from build123d import *

# Parameters (mm, degrees)
ESBO_O1_R                = 62.5
ESBO_O1_R_2              = 4
RESSALTO_EXTRUS_O1_DEPTH = 20
ESBO_O2_R                = 38
RESSALTO_EXTRUS_O2_DEPTH = 35
ESBO_O4_R                = 12
CORTE_EXTRUS_O1_DEPTH    = 25


with BuildPart() as part:
    # Esboço1 → Ressalto-extrusão1 (new body)
    with BuildSketch(Plane(origin=(0, 0, 0), x_dir=(0, 0, -1), z_dir=(1, 0, 0))):
        Circle(ESBO_O1_R)
        with Locations((37.775, 30)):
            Circle(ESBO_O1_R_2, mode=Mode.SUBTRACT)
        with Locations((-37.775, 30)):
            Circle(ESBO_O1_R_2, mode=Mode.SUBTRACT)
        with Locations((37.775, -30)):
            Circle(ESBO_O1_R_2, mode=Mode.SUBTRACT)
        with Locations((-37.775, -30)):
            Circle(ESBO_O1_R_2, mode=Mode.SUBTRACT)
    extrude(amount=RESSALTO_EXTRUS_O1_DEPTH)

    # Esboço2 → Ressalto-extrusão2 (add)
    with BuildSketch(Plane(origin=(20, 0, 0), x_dir=(0, 0, -1), z_dir=(1, 0, 0))):
        Circle(ESBO_O2_R)
    extrude(amount=RESSALTO_EXTRUS_O2_DEPTH)

    # Esboço4 → Corte-extrusão1 (cut)
    with BuildSketch(Plane(origin=(55, 0, 0), x_dir=(0, 0, -1), z_dir=(1, 0, 0))):
        Circle(ESBO_O4_R)
    extrude(amount=-CORTE_EXTRUS_O1_DEPTH, mode=Mode.SUBTRACT)


solid = part.part
Design review of the part built by this model. Coordinates are the model's own, in mm. A direction names the side the tool comes from. Round coordinates to 2 decimals unless told otherwise and drop trailing zeros. Write each loop counter-clockwise with the first axis right and the second up, starting at its lowest first coordinate (ties: lowest second). Pieces come first, ordered by that corner, then holes.
Item 1: For pin 1 Ø5 at (x, z) = (43.5, -16.5) entering from +Y; pin 2 Ø3 at (x, z) = (41.5, -19.5) entering from -Y; pin 3 Ø10.5 at (y, z) = (30, 37.775) entering from +X; pin 4 Ø5 at (y, z) = (-30, -37.775) entering from +X, all flat-tipped, find the tip position at first contact; note any pin that passes through.
Item 2: Consider section B-B on z = 36.5. Give the boundary of the cut face in (x, y).
Item 3: Draft analysis for pull direction Y (two halves, no side actions). For faces 1 (the cylindrical face through (37.255, -33.713, -17.535)), 2 (the flat face through (55, 9, 9)), 3 (the cylindrical face through (9.86, -26.63, -39.93)), state which applies: released by +Y, released by -Y, zero draft, split by the parting line, or undercut.
Item 4: Consider section C-C on x = 13. Give the boundary of the cut face in (y, z) (3 decimals).
Item 5: Consider section A-A on y = 0. Give the boundary of the cut face in (x, z).
Item 6: Consider section D-D on y = -30. Give the boundary of the cut face in (x, z) (3 decimals), and give its area (3 significant figures).
Item 7: Wall thickness on L1, parallel to X at y = -17, z = 39; L2, parallel to X at y = -3, z = 8; L3, parallel to Y at x = 14.5, z = -1: over which ranges is each line inside the solid? List them lowest first.
Item 8: For faces 4 (the flat face through (30, 0, 0)), 5 (the cylindrical face through (9.86, -27.297, 40.723)), list the 3-axis set-ups (+Z, -Z, +X, -X, +Y, -Y) from which the entire face can be reached by the end or side of a thin tool; tool diameter is ignored.
Check values:
1. pin 1: stops at y = 35.33
1. pin 2: stops at y = -33.47
1. pin 3: stops at x = 20
1. pin 4: passes through
2. outline: (0, -50.73) - (20, -50.73) - (20, -33.79) - (0, -33.79) - close; (0, -26.21) - (20, -26.21) - (20, -10.57) - (55, -10.57) - (55, 10.57) - (20, 10.57) - (20, 26.21) - (0, 26.21) - close; (0, 33.79) - (20, 33.79) - (20, 50.73) - (0, 50.73) - close
3. face 1: split by the parting line
3. face 2: zero draft
3. face 3: undercut
4. outline: circle Ø125 at (0, 0); hole circle Ø8 at (-30, -37.775); hole circle Ø8 at (-30, 37.775); hole circle Ø8 at (30, -37.775); hole circle Ø8 at (30, 37.775)
5. outline: (0, -62.5) - (20, -62.5) - (20, -38) - (55, -38) - (55, -12) - (30, -12) - (30, 12) - (55, 12) - (55, 38) - (20, 38) - (20, 62.5) - (0, 62.5) - close
6. outline: (0, -54.829) - (20, -54.829) - (20, -41.775) - (0, -41.775) - close; (0, -33.775) - (20, -33.775) - (20, -23.324) - (55, -23.324) - (55, 23.324) - (20, 23.324) - (20, 33.775) - (0, 33.775) - close; (0, 41.775) - (20, 41.775) - (20, 54.829) - (0, 54.829) - close
6. area: 3,510 mm2
7. L1: x = 0 to 20
7. L2: x = 0 to 30
7. L3: y = -62.49 to 62.49
8. face 4: +X
8. face 5: +X, -X
